Geometry check sheet. Reference: the model listing, model coordinates, mm. A direction names the side the tool comes from. Coordinates: 2 decimals unless noted, no trailing zeros. Order: outer loops, then holes, each group sorted by start corner. A loop starts at its lowest first (then second) coordinate and runs counter-clockwise, first axis right, second up. Notation, with made-up numbers: (18.5, 84) - (77.5, 84) arc R20 ccw to (77.5, 99) - close; hole circle Ø5 at (-26, 72). An arc over 180 degrees is marked (long way). Use CSV: the item, a comma, the result in double quotes. Start each with the question number.
1) Depth check by flat-ended pin: P1, Ø1.6, axis at x = -22, z = 1, coming from the +Y side; P2, Ø1.1, axis at y = 14, z = 2, coming from the -X side; P3, Ø1.6, axis at x = 53.5, z = 1.5, coming from the +Y side. Enter the tip coordinate at first touch or a pass-through.
2) Sectioned sample at A-A, the plane y = -49.5. Record the cut outline in (x, z) (3 decimals).
3) Sectioned sample at D-D, the plane y = -26.5. Record the cut outline in (x, z) (3 decimals).
4) Sectioned sample at B-B, the plane x = -27. Count the separate pieces of the cut face and the enclosed holes in it, and give its area (3 significant figures).
5) Thickness scan on probe 1 along Y at (x, z) = (-29, 2.25) (3 decimals); probe 2 along X at (y, z) = (-13.5, 1.25); probe 3 along Y at (x, z) = (-62, 1.35). Record the ranges inside material, lowest first. Write a range as [from, to].
6) Tool access check on faces 3 (the flat face through (53.4, 6.36, 1.57)), 4 (the flat face through (-73.61, 43.84, 1.57)), 5 (the flat face through (0, 0, 3.175)). Record the directions out of +Z, -Z, +X, -X, +Y, -Y that give a thin tool (end or side, any length) a straight path to the whole face; none if there is none.
7) Draft check along Y on faces 1 (the flat face through (69.426, 51.504, 1.565)), 2 (the flat face through (0, 0, 0)). Enter one of: released by +Y, released by -Y, zero draft, split by the parting line, or undercut.
from build123d import *

# Parameters (mm, degrees)
BOSS_EXTRUDE1_DEPTH = 3.175
SKETCH6_R           = 7.257154646
CUT_EXTRUDE5_DEPTH  = 3.175
SKETCH9_W           = 3.175
SKETCH9_H           = 3.175
CUT_EXTRUDE7_DEPTH  = 3.175
SKETCH8_W           = 30.724562626
SKETCH8_H           = 2.108548415
SKETCH8_H_2         = 2.108548416
CUT_EXTRUDE6_DEPTH  = 3.175
SKETCH10_W          = 20.32
SKETCH10_H          = 3.175
BOSS_EXTRUDE2_DEPTH = 3.175
CUT_EXTRUDE8_DEPTH  = 3.175


with BuildPart() as part:
    # Sketch1 → Boss-Extrude1 (new body)
    with BuildSketch(Plane.XY):
        with BuildLine():
            Line((41.839101774, 27.787790455), (102.197242912, 60.347139319))
            add(Edge.make_bspline(
                [(102.197242912, 60.347139319), (60.742723961, 54.966910385), (20.07049128, 45.384405553)],
                knots=[0, 0, 0, 1, 1, 1], degree=2))
            Line((20.07049128, 45.384405553), (-1.005398806, 45.384405553))
            Line((-1.005398806, 45.384405553), (-1.005398806, -59.17809155))
            Line((-1.005398806, -59.17809155), (62.494601194, -59.17809155))
            ThreePointArc((62.494601194, -59.17809155), (75.141770938, -38.057520175), (50.68909305, -35.212176281))
            Line((50.68909305, -35.212176281), (64.64061298, -14.48138505))
            Line((64.64061298, -14.48138505), (41.839101774, 27.787790455))
        make_face()
    boss_extrude1 = extrude(amount=BOSS_EXTRUDE1_DEPTH)

    # Sketch6 → Cut-Extrude5 (cut)
    with BuildSketch(Plane.XY):
        with Locations((41.928309242, -10.363128131)):
            Circle(SKETCH6_R)
        Polygon((57.996590192, 48.887210307), (81.18043036, 54.194354442), (58.847058779, 42.146931793), align=None)
        with BuildLine():
            Line((-1.005398806, -4.460766145), (-1.005398806, -20.868472516))
            add(Edge.make_bspline(
                [(-1.005398806, -4.460766145), (0.91009084, -8.087601817), (2.163575929, -6.944318239), (3.759225089, -6.904333812), (6.982497489, -5.965665574), (7.107924345, -4.954032148), (8.383749268, -4.7792984), (8.858412265, -5.597884514), (8.059934477, -7.266476525), (5.387533009, -7.743309848), (2.87598619, -9.738386244), (2.165758509, -12.437670072), (2.502299568, -16.460193064), (0.929673731, -19.700918611), (-1.005398806, -20.868472516)],
                knots=[0, 0, 0, 0, 0.201890753, 0.228999657, 0.271089043, 0.343451588, 0.384030867, 0.405551279, 0.412267992, 0.551583373, 0.622208689, 0.702728492, 0.796795757, 1, 1, 1, 1], degree=3))
        make_face()
    cut_extrude5 = extrude(amount=CUT_EXTRUDE5_DEPTH, mode=Mode.SUBTRACT)

    # Sketch9 → Cut-Extrude7 (cut)
    with BuildSketch(Plane(origin=(0, 0, 0), x_dir=(-1, 0, 0), z_dir=(0, 0, -1))):
        with Locations((-53.287101194, -44.89059155)):
            Rectangle(SKETCH9_W, SKETCH9_H)
    cut_extrude7 = extrude(amount=-CUT_EXTRUDE7_DEPTH, mode=Mode.SUBTRACT)

    # Sketch8 → Cut-Extrude6 (cut)
    with BuildSketch(Plane.XY):
        with Locations((-23.52574119, 20.913238549)):
            Rectangle(SKETCH8_W, SKETCH8_H)
        with Locations((-23.52574119, 14.738203903)):
            Rectangle(SKETCH8_W, SKETCH8_H_2)
        with Locations((-23.52574119, 10.069275269)):
            Rectangle(SKETCH8_W, SKETCH8_H)
        with Locations((-23.52574119, 4.044851224)):
            Rectangle(SKETCH8_W, SKETCH8_H_2)
        with Locations((21.514943577, 4.044851224)):
            Rectangle(SKETCH8_W, SKETCH8_H_2)
        with Locations((21.514943577, 10.069275269)):
            Rectangle(SKETCH8_W, SKETCH8_H)
        with Locations((21.514943577, 14.738203903)):
            Rectangle(SKETCH8_W, SKETCH8_H_2)
        with Locations((21.514943577, 20.913238549)):
            Rectangle(SKETCH8_W, SKETCH8_H)
    cut_extrude6 = extrude(amount=CUT_EXTRUDE6_DEPTH, mode=Mode.SUBTRACT)

    # Mirror4: Boss-Extrude1, Cut-Extrude5, Cut-Extrude7, Cut-Extrude6 across plane
    add(boss_extrude1.mirror(Plane(origin=(-1.005398806, 0, 3.175), x_dir=(0, 0, 1), z_dir=(1, 0, 0))))
    add(cut_extrude5.mirror(Plane(origin=(-1.005398806, 0, 3.175), x_dir=(0, 0, 1), z_dir=(1, 0, 0))), mode=Mode.SUBTRACT)
    add(cut_extrude7.mirror(Plane(origin=(-1.005398806, 0, 3.175), x_dir=(0, 0, 1), z_dir=(1, 0, 0))), mode=Mode.SUBTRACT)
    add(cut_extrude6.mirror(Plane(origin=(-1.005398806, 0, 3.175), x_dir=(0, 0, 1), z_dir=(1, 0, 0))), mode=Mode.SUBTRACT)

    # Sketch10 → Boss-Extrude2 (add)
    with BuildSketch(Plane.XZ.offset(59.17809155)):
        with Locations((-28.945398806, 1.5875)):
            Rectangle(SKETCH10_W, SKETCH10_H)
        with Locations((26.934601194, 1.5875)):
            Rectangle(SKETCH10_W, SKETCH10_H)
    extrude(amount=BOSS_EXTRUDE2_DEPTH)

    # Sketch11 → Cut-Extrude8 (cut)
    with BuildSketch(Plane.XY.offset(3.175)):
        Polygon((-49.087598806, -51.55809155), (-49.087598806, -46.47809155), (-40.832598806, -46.47809155), (-40.832598806, -51.55809155), (-43.194798806, -51.55809155), (-43.194798806, -59.17809155), (-46.725398806, -59.17809155), (-46.725398806, -51.55809155), align=None)
        Polygon((-5.145598806, -51.55809155), (-5.145598806, -46.47809155), (3.109401194, -46.47809155), (3.109401194, -51.55809155), (0.747201194, -51.55809155), (0.747201194, -59.17809155), (-2.783398806, -59.17809155), (-2.783398806, -51.55809155), align=None)
        Polygon((38.821801194, -51.55809155), (38.821801194, -46.47809155), (47.076801194, -46.47809155), (47.076801194, -51.55809155), (44.714601194, -51.55809155), (44.714601194, -59.17809155), (41.184001194, -59.17809155), (41.184001194, -51.55809155), align=None)
    extrude(amount=-CUT_EXTRUDE8_DEPTH, mode=Mode.SUBTRACT)


solid = part.part
Evaluation:
1,P1,"y = 45.55"
1,P2,"x = -51.58"
1,P3,"y = 52.68"
2,outline,"(-77.793, 0) - (-49.088, 0) - (-49.088, 3.175) - (-77.793, 3.175) - close; (-40.833, 0) - (-5.146, 0) - (-5.146, 3.175) - (-40.833, 3.175) - close; (3.109, 0) - (38.822, 0) - (38.822, 3.175) - (3.109, 3.175) - close; (47.077, 0) - (75.783, 0) - (75.783, 3.175) - (47.077, 3.175) - close"
3,outline,"(-58.563, 0) - (56.552, 0) - (56.552, 3.175) - (-58.563, 3.175) - close"
4,separate pieces,"5"
4,enclosed holes,"0"
4,area,"319 mm²"
5,probe 1,"[-62.353, 2.991], [5.099, 9.015], [11.124, 13.684], [15.792, 19.859], [21.968, 46.983]"
5,probe 2,"[-66.12, -50.48], [-37.39, -4.29], [2.28, 35.38], [48.47, 64.11]"
5,probe 3,"[-59.18, -30.02], [-21.39, -5.86], [37.58, 42.76], [49.34, 53.74]"
6,face 3,"+Z, -Z, +X"
6,face 4,"+Z, -Z, -X"
6,face 5,"+Z, +X, -X, +Y, -Y"
7,face 1,"undercut"
7,face 2,"zero draft"
